Source: three-view drawing plus pictorial views. Frame: mm from the lowest corner of the part. A direction names the side the tool comes from. Round coordinates to 2 decimals unless told otherwise and drop trailing zeros. Loops run counter-clockwise (first coordinate to the right, second up) from the corner with the lowest first, then second, coordinate; pieces in that order, holes last. Notation, with made-up numbers: (29, -8) -> (37, -8) arc R21 ccw to (37, 6) -> close; hole circle Ø11 at (-32, -37). An arc over 180 degrees is marked (long way). Put each result on its own line as item: value. Start each with the question number.
1. Cut plane A-A (x = 63). Return the cut outline in (y, z).
2. Set-up query: the marked faces 4, 5 and 6. Return all of +Z, -Z, +X, -X, +Y, -Y with unobstructed straight access to the full face (end or side cutting, diameter ignored); none if empty.
3. Cut plane B-B (z = 94). Return the cut outline in (x, y), then the cut area to 3 significant figures.
4. Draft query along X for the marked faces 1, 2 and 3. Return one class per face: pulls with the +X half, pulls with the -X half, needs draft (parallel to the pull), parting line crosses it, or undercut.
5. Material intervals for L1, parallel to Y at x = 41.5, z = 56.5; L2, parallel to Y at x = 90, z = 51.5; L3, parallel to X at y = 19, z = 45, sorted ascending.
6. Cut plane C-C (y = 21). Return the cut outline in (x, z), then the cut area to 3 significant figures.
7. Cut plane D-D (x = 11). Return the cut outline in (y, z).
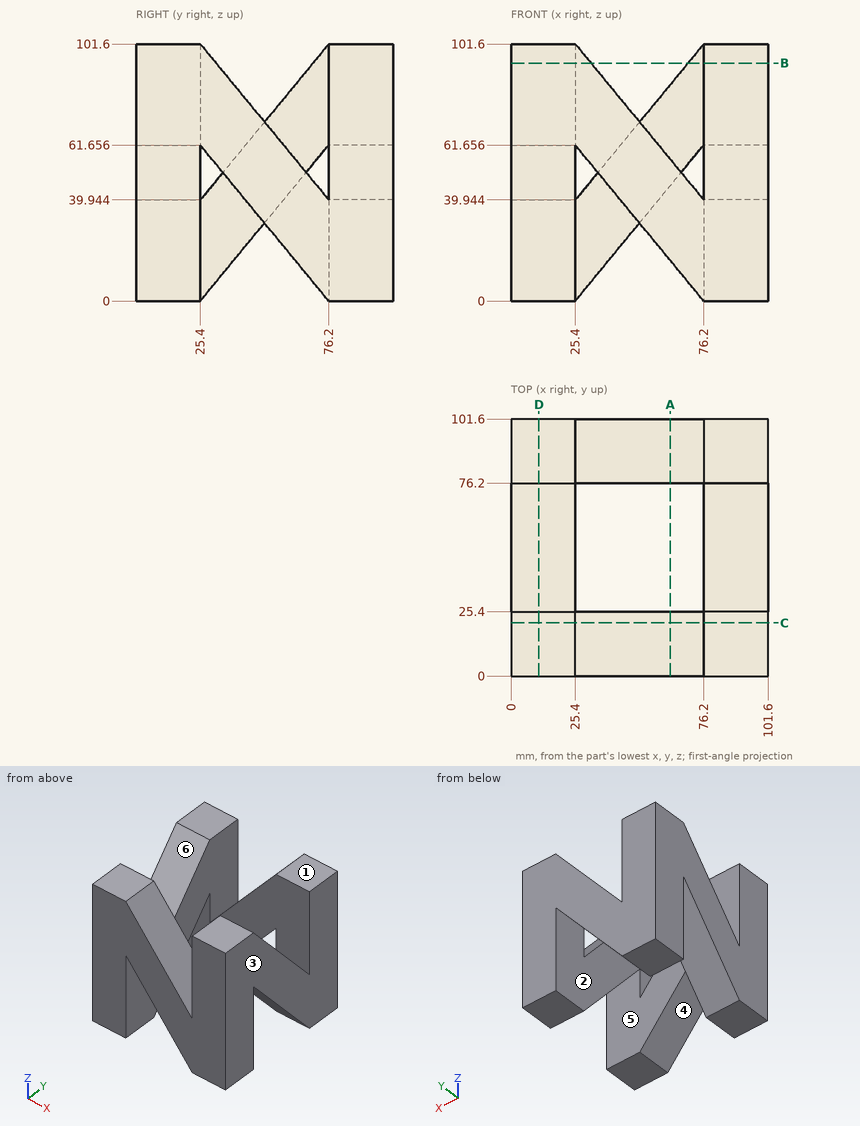
Solution:
1. outline: (0, 16.02) -> (25.4, 16.02) -> (25.4, 55.96) -> (0, 55.96) -> close; (76.2, 45.64) -> (101.6, 45.64) -> (101.6, 85.58) -> (76.2, 85.58) -> close
2. face 4: -Z, -Y
2. face 5: none
2. face 6: +Z, -X
3. outline: (0, 0) -> (31.66, 0) -> (31.66, 25.4) -> (0, 25.4) -> close; (0, 69.94) -> (25.4, 69.94) -> (25.4, 101.6) -> (0, 101.6) -> close; (69.94, 76.2) -> (101.6, 76.2) -> (101.6, 101.6) -> (69.94, 101.6) -> close; (76.2, 0) -> (101.6, 0) -> (101.6, 31.66) -> (76.2, 31.66) -> close
3. area: 3,220 mm^2
4. face 1: needs draft
4. face 2: undercut
4. face 3: pulls with the +X half
5. L1: y = 0 to 25.4, 76.2 to 101.6
5. L2: y = 0 to 25.4, 33.77 to 66.68, 76.2 to 101.6
5. L3: x = 0 to 25.4, 39.12 to 72.03, 76.2 to 101.6
6. outline: (0, 0) -> (25.4, 0) -> (25.4, 61.66) -> (76.2, 0) -> (101.6, 0) -> (101.6, 101.6) -> (76.2, 101.6) -> (76.2, 39.94) -> (25.4, 101.6) -> (0, 101.6) -> close
6. area: 7,190 mm^2
7. outline: (0, 0) -> (25.4, 0) -> (76.2, 61.66) -> (76.2, 0) -> (101.6, 0) -> (101.6, 101.6) -> (76.2, 101.6) -> (25.4, 39.94) -> (25.4, 101.6) -> (0, 101.6) -> close
